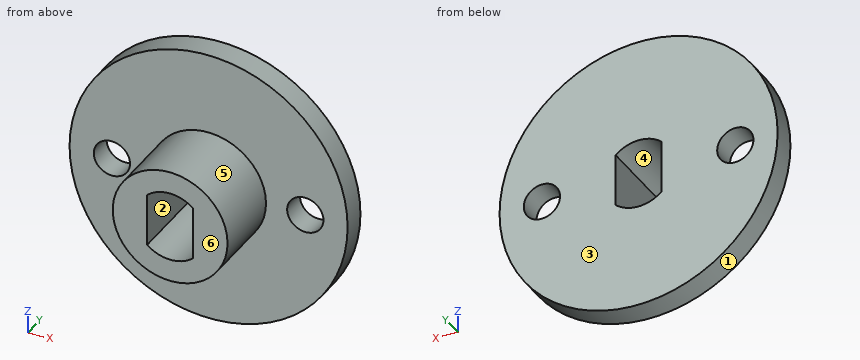
from build123d import *

# Parameters (mm, degrees)
F0_R     = 4.75
F1_DEPTH = 8
F0_R_2   = 11.5
F0_R_3   = 1.5
F2_DEPTH = 2


# Not quite as in the source:
# - a feature names something its author has since deleted; it is built from what else it names


with BuildPart() as f1:
    # F0 (on Front) → F1 (new body)
    with BuildSketch(Plane.XZ):
        Circle(F0_R)
        with BuildLine():
            ThreePointArc((1.9, 2.19089023), (2.6381811917, 1.2041594579), (2.9, 0))
            ThreePointArc((2.9, 0), (2.6381811917, -1.2041594579), (1.9, -2.19089023))
            ThreePointArc((1.9, -2.19089023), (0, -2.9), (-1.9, -2.19089023))
            ThreePointArc((-1.9, -2.19089023), (-2.9, 0), (-1.9, 2.19089023))
            ThreePointArc((-1.9, 2.19089023), (0, 2.9), (1.9, 2.19089023))
        make_face(mode=Mode.SUBTRACT)
        with BuildLine():
            Line((-1.9, -2.19089023), (-1.9, 2.19089023))
            ThreePointArc((-1.9, 2.19089023), (-2.9, 0), (-1.9, -2.19089023))
        make_face()
        with BuildLine():
            ThreePointArc((1.9, -2.19089023), (2.6381811917, -1.2041594579), (2.9, 0))
            ThreePointArc((2.9, 0), (2.6381811917, 1.2041594579), (1.9, 2.19089023))
            Line((1.9, 2.19089023), (1.9, -2.19089023))
        make_face()
    extrude(amount=F1_DEPTH)

    # F0 (on Front) → F2 (join)
    with BuildSketch(Plane.XZ):
        Circle(F0_R_2)
        with Locations((-8, 0)):
            Circle(F0_R_3, mode=Mode.SUBTRACT)
        Circle(F0_R, mode=Mode.SUBTRACT)
        with Locations((8, 0)):
            Circle(F0_R_3, mode=Mode.SUBTRACT)
    extrude(amount=F2_DEPTH)


solid = f1.part
Geometry: final body of the model. Coordinates: model frame, mm. Face numbers are marked on the shaded views. A direction names the side the tool comes from. Give positions to 0.01 mm unless a question says otherwise; leave off trailing zeros. Loops run counter-clockwise (first coordinate to the right, second up) from the corner with the lowest first, then second, coordinate; pieces in that order, holes last. Notation, with made-up numbers: (40.25, 25) - (65.25, 25) arc R22 cw to (65.25, 42) - close; hole circle Ø2 at (52, 4.25). An arc over 180 degrees is marked (long way). Answer as CSV lines item,"result". Start each with the question number.
1. Section C-C, the plane y = -7. Return loops of the section in (x, z), plus the area to 3 significant figures.
2. Ray query, L1, parallel to X at y = -4.75, z = -0.25; L2, parallel to Y at x = -7.25, z = 4.5; L3, parallel to Z at x = 8, y = -0.7. Return the intervals inside material, ascending.
3. Section D-D, the plane x = -8. Return loops of the section in (y, z).
4. Section A-A, the plane x = 0. Return loops of the section in (y, z), plus the area to 3 significant figures.
5. Reachability of the marked faces 4, 5 and 6 from +Z, -Z, +X, -X, +Y, -Y: full face, straight path, thin tool, end or side. Return the list, or none.
6. Draft query along X for the marked faces 1, 2 and 3. Return one class per face: released by +X, released by -X, zero draft, split by the parting line, or undercut.
7. Pin query (flat end, axial travel): P1, Ø1.5, axis at y = -3, z = 1, coming from the -X side; P2, Ø2, axis at x = -8.5, z = -4.5, coming from the -Y side; P3, Ø1.3, axis at y = -4, z = -0.5, coming from the +X side. Return the tip coordinate at first contact, or that it passes through.
8. Section B-B, the plane z = 0. Return loops of the section in (x, y).
Answers:
1,outline,"circle Ø9.5 at (0, 0); hole (-1.9, -2.19) arc R2.9 ccw to (1.9, -2.19) - (1.9, 2.19) arc R2.9 ccw to (-1.9, 2.19) - close"
1,area,"50.5 mm2"
2,L1,"x = -4.74 to -1.9, 1.9 to 4.74"
2,L2,"y = -2 to 0"
2,L3,"z = -8.26 to -1.5, 1.5 to 8.26"
3,outline,"(-2, -8.26) - (0, -8.26) - (0, -1.5) - (-2, -1.5) - close; (-2, 1.5) - (0, 1.5) - (0, 8.26) - (-2, 8.26) - close"
4,outline,"(-8, -4.75) - (-2, -4.75) - (-2, -11.5) - (0, -11.5) - (0, -2.9) - (-8, -2.9) - close; (-8, 2.9) - (0, 2.9) - (0, 11.5) - (-2, 11.5) - (-2, 4.75) - (-8, 4.75) - close"
4,area,"56.6 mm2"
5,face 4,"+Y, -Y"
5,face 5,"-Y"
5,face 6,"+Z, -Z, +X, -X, -Y"
6,face 1,"split by the parting line"
6,face 2,"undercut"
6,face 3,"zero draft"
7,P1,"stops at x = -4.74"
7,P2,"stops at y = -2"
7,P3,"stops at x = 4.75"
8,outline,"(-11.5, -2) - (-9.5, -2) - (-9.5, 0) - (-11.5, 0) - close; (-6.5, -2) - (-4.75, -2) - (-4.75, -8) - (-1.9, -8) - (-1.9, 0) - (-6.5, 0) - close; (1.9, -8) - (4.75, -8) - (4.75, -2) - (6.5, -2) - (6.5, 0) - (1.9, 0) - close; (9.5, -2) - (11.5, -2) - (11.5, 0) - (9.5, 0) - close"
